Source: CAD feature listing. Evaluate the final solid. Frame: model axes, mm. A direction names the side the tool comes from. Give positions to 0.01 mm unless a question says otherwise; leave off trailing zeros. Loops run counter-clockwise (first coordinate to the right, second up) from the corner with the lowest first, then second, coordinate; pieces in that order, holes last.
from build123d import *

# Parameters (mm, degrees)
SKETCH1_W           = 55
SKETCH1_H           = 14
BOSS_EXTRUDE1_DEPTH = 5.715
SKETCH2_R           = 1.75
CUT_EXTRUDE1_DEPTH  = 52.394687241
SKETCH3_W           = 31
SKETCH3_H           = 5.715
BOSS_EXTRUDE2_DEPTH = 31
SKETCH4_R           = 1.55
CUT_EXTRUDE2_DEPTH  = 84.264914302
FILLET1_R           = 2


with BuildPart() as part:
    # Sketch1 → Boss-Extrude1 (new body)
    with BuildSketch(Plane(origin=(0, 0, 0), x_dir=(1, 0, 0), z_dir=(0, 1, 0))):
        with Locations((23.05007671, 0.310430648)):
            Rectangle(SKETCH1_W, SKETCH1_H)
    extrude(amount=BOSS_EXTRUDE1_DEPTH)

    # Sketch2 → Cut-Extrude1 (cut, through all)
    with BuildSketch(Plane(origin=(0, 5.715, 0), x_dir=(1, 0, 0), z_dir=(0, 1, 0))):
        with Locations(Location((8.55007671, 0.310430648, 0), (0, 0, 270))):
            Circle(SKETCH2_R)
        with Locations(Location((36.55007671, 0.310430648, 0), (0, 0, 270))):
            Circle(SKETCH2_R)
    extrude(amount=-CUT_EXTRUDE1_DEPTH, mode=Mode.SUBTRACT)

    # Sketch3 → Boss-Extrude2 (add)
    with BuildSketch(Plane(origin=(50.55007671, 0, 0), x_dir=(0, 0, -1), z_dir=(1, 0, 0))):
        with Locations((0.310430648, 2.8575)):
            Rectangle(SKETCH3_W, SKETCH3_H)
    extrude(amount=BOSS_EXTRUDE2_DEPTH)

    # Sketch4 → Cut-Extrude2 (cut, through all)
    with BuildSketch(Plane(origin=(0, 5.715, 0), x_dir=(1, 0, 0), z_dir=(0, 1, 0))):
        with Locations(Location((57.211241945, -8.838834765, 0), (0, 0, 270))):
            Circle(SKETCH4_R)
        with Locations(Location((59.438628306, 6.611448404, 0), (0, 0, 270))):
            Circle(SKETCH4_R)
        with Locations(Location((74.888911475, 8.838834765, 0), (0, 0, 270))):
            Circle(SKETCH4_R)
        with Locations(Location((72.661525114, -6.611448404, 0), (0, 0, 270))):
            Circle(SKETCH4_R)
    extrude(amount=-CUT_EXTRUDE2_DEPTH, mode=Mode.SUBTRACT)

    # Fillet1
    fillet1_edges = [part.edges().sort_by_distance(p)[0] for p in [
        (-4.44992329, 2.8575, -7.310430648),
        (-4.44992329, 2.8575, 6.689569352),
        (50.55007671, 2.8575, -7.310430648),
        (50.55007671, 2.8575, 6.689569352),
        (50.55007671, 2.8575, -15.810430648),
        (81.55007671, 2.8575, -15.810430648),
        (81.55007671, 2.8575, 15.189569352),
        (50.55007671, 2.8575, 15.189569352),
    ]]
    fillet(fillet1_edges, radius=FILLET1_R)


solid = part.part
1) Contact query for flat-ended pins moving along their axis: P1, Ø3.5, axis at x = 59.44, z = -6.61, coming from the +Y side (3 decimals); P2, Ø1.3, axis at y = 2.5, z = 10, coming from the -X side; P3, Ø2, axis at y = 5, z = 8.5, coming from the -X side; P4, Ø3, axis at x = 33.5, y = 3, coming from the +Z side. Output: stop coordinate, or through.
Checks:
P1: stops at y = 5.715
P2: stops at x = 50.55
P3: stops at x = 50.16
P4: stops at z = 6.69
2) Reachability of faces 1 (the flat face through (48, 5.715, 0)), 2 (the flat face through (23, 3, 6.69)) from +Z, -Z, +X, -X, +Y, -Y: full face, straight path, thin tool, end or side. Return the list, or none.
Checks:
face 1: +Z, -Z, +X, -X, +Y
face 2: +Z, -X, +Y, -Y
3) Cut plane C-C (x = 17.5). Return loops of the section in (y, z) (3 decimals).
Checks:
outline: (0, -7.31) - (5.715, -7.31) - (5.715, 6.69) - (0, 6.69) - close
4) Cut plane A-A (z = -1). Return loops of the section in (x, y) (1 decimal), and give its area (3 significant figures).
Checks:
outline: (-4.4, 0) - (6.9, 0) - (6.9, 5.7) - (-4.4, 5.7) - close; (10.2, 0) - (34.9, 0) - (34.9, 5.7) - (10.2, 5.7) - close; (38.2, 0) - (81.6, 0) - (81.6, 5.7) - (38.2, 5.7) - close
area: 455 mm2
5) Pull-direction query (X, two-part tool) for faces 3 (the cylindrical face through (74.2, 2.9, 6.41)), 4 (the flat face through (48, 0, 0)), 5 (the flat face through (81.55, 3, 0)), 6 (the cylindrical face through (55.7, 2.9, 8.5)); classes: released by +X, released by -X, zero draft, split by the parting line, or undercut.
Checks:
face 3: undercut
face 4: zero draft
face 5: released by +X
face 6: undercut
6) Ray query, probe 1 along X at (y, z) = (3.1, -0.5); probe 2 along Z at (x, y) = (59.5, 2); probe 3 along Z at (x, y) = (42, 0.4). Return the intervals inside material, ascending.
Checks:
probe 1: x = -4.45 to 6.81, 10.29 to 34.81, 38.29 to 81.55
probe 2: z = -15.81 to -8.16, -5.06 to 15.19
probe 3: z = -7.31 to 6.69
7) Cut plane B-B (y = 4.85). Return loops of the section in (x, z), and give its area (3 significant figures).
Checks:
outline: (-4.45, -5.31) arc R2 ccw to (-2.45, -7.31) - (48.55, -7.31) arc R2 cw to (50.55, -9.31) - (50.55, -13.81) arc R2 ccw to (52.55, -15.81) - (79.55, -15.81) arc R2 ccw to (81.55, -13.81) - (81.55, 13.19) arc R2 ccw to (79.55, 15.19) - (52.55, 15.19) arc R2 ccw to (50.55, 13.19) - (50.55, 8.69) arc R2 cw to (48.55, 6.69) - (-2.45, 6.69) arc R2 ccw to (-4.45, 4.69) - close; hole circle Ø3.5 at (8.55, -0.31); hole circle Ø3.5 at (36.55, -0.31); hole circle Ø3.1 at (57.21, 8.84); hole circle Ø3.1 at (59.44, -6.61); hole circle Ø3.1 at (72.66, 6.61); hole circle Ø3.1 at (74.89, -8.84)
area: 1,680 mm2
